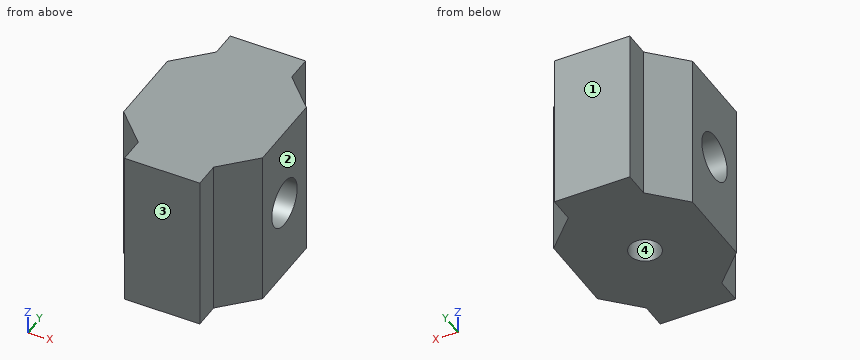
from build123d import *

# Parameters (mm, degrees)
BOSS_EXTRUDE1_DEPTH     = 20
SKETCH2_R               = 3
CUT_EXTRUDE1_DEPTH      = 20
CUT_EXTRUDE1_DEPTH_BACK = 20
SKETCH3_R               = 1.95
CUT_EXTRUDE2_DEPTH      = 6


with BuildPart() as part:
    # Sketch1 → Boss-Extrude1 (new body)
    with BuildSketch(Plane.XY):
        Polygon((4.772, -12.514), (4.772, -9.231678019), (8.8, -5.167678019), (8.8, 0), (8.8, 5.167678019), (4.772, 9.231678019), (4.772, 12.514), (-4.772, 12.514), (-4.772, 9.231678019), (-8.8, 5.167678019), (-8.8, 0), (-8.8, -5.167678019), (-4.772, -9.231678019), (-4.772, -12.514), align=None)
    extrude(amount=BOSS_EXTRUDE1_DEPTH)

    # Sketch2 → Cut-Extrude1 (cut, two sides)
    with BuildSketch(Plane(origin=(0, 0, 0), x_dir=(0, 0, -1), z_dir=(1, 0, 0))) as cut_extrude1_sk:
        with Locations((-10, 0)):
            Circle(SKETCH2_R)
    extrude(amount=CUT_EXTRUDE1_DEPTH, mode=Mode.SUBTRACT)
    extrude(cut_extrude1_sk.sketch, amount=-CUT_EXTRUDE1_DEPTH_BACK, mode=Mode.SUBTRACT)

    # Sketch3 → Cut-Extrude2 (cut)
    with BuildSketch(Plane(origin=(0, 0, 0), x_dir=(-1, 0, 0), z_dir=(0, 0, -1))):
        Circle(SKETCH3_R)
    extrude(amount=-CUT_EXTRUDE2_DEPTH, mode=Mode.SUBTRACT)


solid = part.part
Could you check a few things on this model? Use its own coordinates, in mm. Face numbers are marked on the shaded views. Round coordinates to 2 decimals unless told otherwise and drop trailing zeros. Write each loop counter-clockwise with the first axis right and the second up, starting at its lowest first coordinate (ties: lowest second). Pieces come first, ordered by that corner, then holes. Notation, with made-up numbers: (-29, 4) -> (16, 4) arc R28 ccw to (16, 37) -> close; hole circle Ø8 at (-23, 4.5). An arc over 180 degrees is marked (long way). Use a Markdown table: item, result.
1. For pin 1 Ø3 at (x, y) = (0, 0) entering from -Z; pin 2 Ø5 at (y, z) = (10, 16) entering from +X; pin 3 Ø3 at (y, z) = (9.5, 2) entering from +X, each with a flat end and sliding along its axis, tell me the tip position at first contact or that it passes through.
Answer key:
| item | result |
|---|---|
| pin 1 | stops at z = 6 |
| pin 2 | stops at x = 6.49 |
| pin 3 | stops at x = 5.99 |
2. If we section it at A-A (z = 2.25): List the corners of the cut face in (x, y) for me, then the cut area to 3 significant figures.
Answer key:
| item | result |
|---|---|
| outline | (-8.8, -5.17) -> (-4.77, -9.23) -> (-4.77, -12.51) -> (4.77, -12.51) -> (4.77, -9.23) -> (8.8, -5.17) -> (8.8, 5.17) -> (4.77, 9.23) -> (4.77, 12.51) -> (-4.77, 12.51) -> (-4.77, 9.23) -> (-8.8, 5.17) -> close; hole circle Ø3.9 at (0, 0) |
| area | 343 mm^2 |
3. Please list where these lines run through material, in increasing order: probe 1 along Z at (x, y) = (6.25, 0); probe 2 along Y at (x, z) = (3.5, 10); probe 3 along Y at (x, z) = (0, 2.85).
Answer key:
| item | result |
|---|---|
| probe 1 | z = 0 to 7, 13 to 20 |
| probe 2 | y = -12.51 to -3, 3 to 12.51 |
| probe 3 | y = -12.51 to -1.95, 1.95 to 12.51 |
4. If we section it at B-B (y = 0): List the corners of the cut face in (x, z) for me.
Answer key:
| item | result |
|---|---|
| outline | (-8.8, 0) -> (-1.95, 0) -> (-1.95, 6) -> (1.95, 6) -> (1.95, 0) -> (8.8, 0) -> (8.8, 7) -> (-8.8, 7) -> close; (-8.8, 13) -> (8.8, 13) -> (8.8, 20) -> (-8.8, 20) -> close |
5. If we section it at C-C (z = 10): List the corners of the cut face in (x, y) for me, then the cut area to 3 significant figures.
Answer key:
| item | result |
|---|---|
| outline | (-8.8, -5.17) -> (-4.77, -9.23) -> (-4.77, -12.51) -> (4.77, -12.51) -> (4.77, -9.23) -> (8.8, -5.17) -> (8.8, -3) -> (-8.8, -3) -> close; (-8.8, 3) -> (8.8, 3) -> (8.8, 5.17) -> (4.77, 9.23) -> (4.77, 12.51) -> (-4.77, 12.51) -> (-4.77, 9.23) -> (-8.8, 5.17) -> close |
| area | 249 mm^2 |
6. We'd pull the mould along Y, two halves only. Please class the marked faces 1, 2, 3 and 4: +Y half, -Y half, draft (parallel to the pull), parting line (faces both ways), or undercut.
Answer key:
| item | result |
|---|---|
| face 1 | +Y half |
| face 2 | draft |
| face 3 | -Y half |
| face 4 | undercut |
7. If we section it at D-D (z = 16): List the corners of the cut face in (x, y) for me.
Answer key:
| item | result |
|---|---|
| outline | (-8.8, -5.17) -> (-4.77, -9.23) -> (-4.77, -12.51) -> (4.77, -12.51) -> (4.77, -9.23) -> (8.8, -5.17) -> (8.8, 5.17) -> (4.77, 9.23) -> (4.77, 12.51) -> (-4.77, 12.51) -> (-4.77, 9.23) -> (-8.8, 5.17) -> close |
